Geometry: final body of the model. Coordinates: model frame, mm. A direction names the side the tool comes from. Give positions to 0.01 mm unless a question says otherwise; leave off trailing zeros. Write each loop counter-clockwise with the first axis right and the second up, starting at its lowest first coordinate (ties: lowest second). Pieces come first, ordered by that corner, then holes. Notation, with made-up numbers: (-28.5, -31) - (8.5, -31) arc R23 cw to (8.5, -20) - close; hole circle Ø11 at (-20.75, -37.5). An arc over 180 degrees is marked (long way). Return JSON: item names as keys, results as strings.
from build123d import *

# Parameters (mm, degrees)
BOSS_EXTRUDE1_DEPTH = 0.508
SKETCH2_R           = 7.874
SKETCH2_R_2         = 6.35
CUT_EXTRUDE2_DEPTH  = 0.254
SKETCH5_R           = 6.354160617
CUT_EXTRUDE3_DEPTH  = 68.821805137
SKETCH6_R           = 5.461
CUT_EXTRUDE4_DEPTH  = 68.821805137
SKETCH7_W           = 19.558
SKETCH7_H           = 1.016
CUT_EXTRUDE5_DEPTH  = 68.823232008
SKETCH8_W           = 6.35
SKETCH8_H           = 0.254
BOSS_EXTRUDE2_DEPTH = 2.032
SKETCH10_W          = 11.303182767
SKETCH10_H          = 0.254
BOSS_EXTRUDE3_DEPTH = 2.032
SKETCH11_W          = 6.35
SKETCH11_H          = 0.254
BOSS_EXTRUDE4_DEPTH = 2.032
SKETCH12_W          = 11.938
SKETCH12_H          = 0.254
BOSS_EXTRUDE5_DEPTH = 2.032
SKETCH13_R          = 7.874
CUT_EXTRUDE7_DEPTH  = 0.254
SKETCH14_R          = 7.874
SKETCH14_R_2        = 5.461
BOSS_EXTRUDE8_DEPTH = 0.254


with BuildPart() as part:
    # Sketch1 → Boss-Extrude1 (new body)
    with BuildSketch(Plane.XY):
        with BuildLine():
            ThreePointArc((0, -10.16), (10.16, 0), (0, 10.16))
            Line((0, 10.16), (-67.056, 10.16))
            Line((-67.056, 10.16), (-67.056, -10.16))
            Line((-67.056, -10.16), (0, -10.16))
        make_face()
    extrude(amount=BOSS_EXTRUDE1_DEPTH)

    # Sketch2 → Cut-Extrude2 (cut)
    with BuildSketch(Plane.XY.offset(0.508)):
        with Locations((-54.61, 0)):
            Circle(SKETCH2_R)
        with Locations((-35.814, 0)):
            Circle(SKETCH2_R_2)
    extrude(amount=-CUT_EXTRUDE2_DEPTH, mode=Mode.SUBTRACT)

    # Sketch5 → Cut-Extrude3 (cut, through all)
    with BuildSketch(Plane.XY.offset(0.254)):
        with Locations((-35.814, 0)):
            Circle(SKETCH5_R)
    extrude(amount=-CUT_EXTRUDE3_DEPTH, mode=Mode.SUBTRACT)

    # Sketch6 → Cut-Extrude4 (cut, through all)
    with BuildSketch(Plane.XY.offset(0.254)):
        with Locations((-54.61, 0)):
            Circle(SKETCH6_R)
    extrude(amount=-CUT_EXTRUDE4_DEPTH, mode=Mode.SUBTRACT)

    # Sketch7 → Cut-Extrude5 (cut, through all)
    with BuildSketch(Plane(origin=(0, 0, 0), x_dir=(-1, 0, 0), z_dir=(0, 0, -1))):
        with Locations((50.927, 9.652)):
            Rectangle(SKETCH7_W, SKETCH7_H)
        with Locations((50.927, -9.652)):
            Rectangle(SKETCH7_W, SKETCH7_H)
    extrude(amount=-CUT_EXTRUDE5_DEPTH, mode=Mode.SUBTRACT)

    # Sketch8 → Boss-Extrude2 (add)
    with BuildSketch(Plane(origin=(0, 0, 0), x_dir=(-1, 0, 0), z_dir=(0, 0, -1))):
        with Locations((63.881, 10.033)):
            Rectangle(SKETCH8_W, SKETCH8_H)
    extrude(amount=BOSS_EXTRUDE2_DEPTH)

    # Sketch10 → Boss-Extrude3 (add)
    with BuildSketch(Plane(origin=(0, 0, 0), x_dir=(-1, 0, 0), z_dir=(0, 0, -1))):
        with Locations((35.496408617, 10.033)):
            Rectangle(SKETCH10_W, SKETCH10_H)
    extrude(amount=BOSS_EXTRUDE3_DEPTH)

    # Sketch11 → Boss-Extrude4 (add)
    with BuildSketch(Plane(origin=(0, 0, 0), x_dir=(-1, 0, 0), z_dir=(0, 0, -1))):
        with Locations((63.881, -10.033)):
            Rectangle(SKETCH11_W, SKETCH11_H)
    extrude(amount=BOSS_EXTRUDE4_DEPTH)

    # Sketch12 → Boss-Extrude5 (add)
    with BuildSketch(Plane(origin=(0, 0, 0), x_dir=(-1, 0, 0), z_dir=(0, 0, -1))):
        with Locations((35.179, -10.033)):
            Rectangle(SKETCH12_W, SKETCH12_H)
    extrude(amount=BOSS_EXTRUDE5_DEPTH)

    # Sketch13 → Cut-Extrude7 (cut)
    with BuildSketch(Plane.XY.offset(0.508)):
        with Locations((-35.814, 0)):
            Circle(SKETCH13_R)
    extrude(amount=-CUT_EXTRUDE7_DEPTH, mode=Mode.SUBTRACT)

    # Sketch14 → Boss-Extrude8 (add)
    with BuildSketch(Plane.XY.offset(0.508)):
        with Locations((-54.61, 0)):
            Circle(SKETCH14_R)
        with Locations((-54.61, 0)):
            Circle(SKETCH14_R_2, mode=Mode.SUBTRACT)
    extrude(amount=-BOSS_EXTRUDE8_DEPTH)


solid = part.part
Q1. Material intervals for probe 1 along Y at (x, z) = (-54.61, 0.2); probe 2 along Y at (x, z) = (-61, -1.75); probe 3 along Z at (x, y) = (-32, -8.5), sorted ascending. Write a range as [from, to].
Answer key:
{"probe 1": "y = [-9.14, -5.46], [5.46, 9.14]", "probe 2": "y = [-10.16, -9.91], [9.91, 10.16]", "probe 3": "z = [0, 0.51]"}
Q2. Section query C-C, the plane y = -4. Return the cut outline in (x, z), plus the area to 3 significant figures.
Answer key:
{"outline": "(-67.06, 0) - (-58.33, 0) - (-58.33, 0.51) - (-67.06, 0.51) - close; (-50.89, 0) - (-40.75, 0) - (-40.75, 0.25) - (-42.6, 0.25) - (-42.6, 0.51) - (-50.89, 0.51) - close; (-30.88, 0) - (9.34, 0) - (9.34, 0.51) - (-29.03, 0.51) - (-29.03, 0.25) - (-30.88, 0.25) - close", "area": "29.1 mm^2"}
Q3. Set-up query: faces 1 (the flat face through (-41, 4, 0.254)), 2 (the flat face through (-64, -10.16, -1)), 3 (the flat face through (-35, -9.906, -1)). Return all of +Z, -Z, +X, -X, +Y, -Y with unobstructed straight access to the full face (end or side cutting, diameter ignored); none if empty.
Answer key:
{"face 1": "+Z", "face 2": "+Z, -Z, +X, -X, -Y", "face 3": "-Z, +X, -X"}
Q4. Pin query (flat end, axial travel): P1, Ø6, axis at x = -45.5, y = -7, coming from the -Z side; P2, Ø0.6, axis at x = -55, z = 0, coming from the +Y side; P3, Ø1, axis at x = 1.5, z = 0, coming from the -Y side. Return the tip coordinate at first contact, or that it passes through.
Answer key:
{"P1": "stops at z = 0", "P2": "stops at y = 9.14", "P3": "stops at y = -10.11"}
Q5. Section query A-A, the plane y = 0. Return the cut outline in (x, z), plus the area to 3 significant figures.
Answer key:
{"outline": "(-67.06, 0) - (-60.07, 0) - (-60.07, 0.51) - (-67.06, 0.51) - close; (-49.15, 0) - (-42.17, 0) - (-42.17, 0.25) - (-43.69, 0.25) - (-43.69, 0.51) - (-49.15, 0.51) - close; (-29.46, 0) - (10.16, 0) - (10.16, 0.51) - (-27.94, 0.51) - (-27.94, 0.25) - (-29.46, 0.25) - close", "area": "26.4 mm^2"}
Q6. Section query D-D, the plane x = -4. Return the cut outline in (y, z).
Answer key:
{"outline": "(-10.16, 0) - (10.16, 0) - (10.16, 0.51) - (-10.16, 0.51) - close"}
Q7. Mould query, pull axis X, two halves, no side actions, for faces 4 (the flat face through (-67.056, 0, 0.3)), 5 (the cylindrical face through (10.158, -0.223, 0.25)), 6 (the cylindrical face through (-58.635, 3.691, 0.258)), 7 (the flat face through (-34, 10.16, 0)). Classes: pulls with the +X half, pulls with the -X half, needs draft (parallel to the pull), parting line crosses it, or undercut.
Answer key:
{"face 4": "pulls with the -X half", "face 5": "pulls with the +X half", "face 6": "undercut", "face 7": "needs draft"}
Q8. Section query B-B, the plane x = -54.61. Return the cut outline in (y, z).
Answer key:
{"outline": "(-9.14, 0) - (-5.46, 0) - (-5.46, 0.51) - (-9.14, 0.51) - close; (5.46, 0) - (9.14, 0) - (9.14, 0.51) - (5.46, 0.51) - close"}
